from build123d import *

# Parameters (mm, degrees)
F0_R     = 12.5
F1_DEPTH = 6.5
F2_R     = 10
F3_DEPTH = 5
F4_R     = 8
F5_DEPTH = 11.501
F6_SIZE  = 0.2


with BuildPart() as f1:
    # F0 (on Top) → F1 (new body)
    with BuildSketch(Plane.XY):
        Circle(F0_R)
    extrude(amount=F1_DEPTH)

    # F2 (on face) → F3 (join)
    with BuildSketch(Plane.XY.offset(6.5)):
        Circle(F2_R)
    extrude(amount=F3_DEPTH)

    # F4 (on face) → F5 (cut, through all)
    with BuildSketch(Plane.XY.offset(11.5)):
        Circle(F4_R)
    extrude(amount=-F5_DEPTH, mode=Mode.SUBTRACT)

    # F6
    f6_edges = [f1.edges().sort_by_distance(p)[0] for p in [
        (-10, 0, 11.5),
        (-8, 0, 11.5),
        (-12.5, 0, 6.5),
        (-10, 0, 6.5),
        (-12.5, 0, 0),
        (-8, 0, 0),
    ]]
    chamfer(f6_edges, length=F6_SIZE)


solid = f1.part
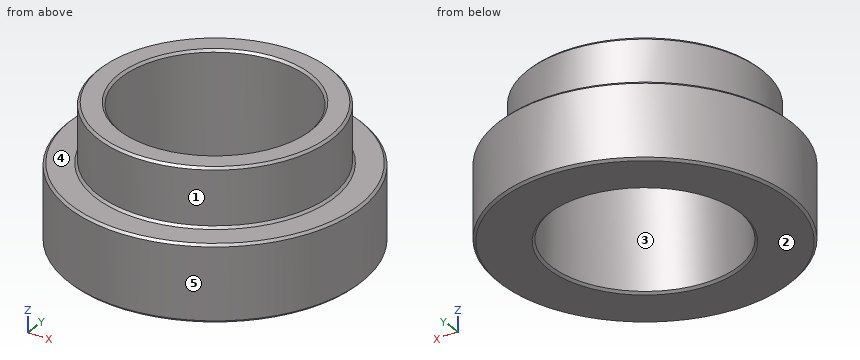
For this review, take the finished solid that the model builds, in its own axes (mm). Face numbers are marked on the shaded views. A direction names the side the tool comes from. Round coordinates to 2 decimals unless told otherwise and drop trailing zeros. Loops run counter-clockwise (first coordinate to the right, second up) from the corner with the lowest first, then second, coordinate; pieces in that order, holes last. Notation, with made-up numbers: (71.25, 22.25) - (81.25, 22.25) arc R8 ccw to (81.25, 36.25) - close; hole circle Ø11 at (-19.75, -23). An arc over 180 degrees is marked (long way). One line per item, written item: value. Start each with the question number.
Item 1: Take a section at C-C (z = 8). Give the boundary of the cut face in (x, y), plus the area to 3 significant figures.
Item 2: For the marked faces 1 and 2, list the 3-axis set-ups (+Z, -Z, +X, -X, +Y, -Y) from which the entire face can be reached by the end or side of a thin tool; tool diameter is ignored.
Item 3: For L1, parallel to Y at x = 0, z = 7; L2, parallel to Y at x = 0, z = 6.25; L3, parallel to Z at x = 8.75, y = 5.5, list the stretches that pass through material, from the lowest coordinate up.
Item 4: Take a section at D-D (z = 2.5). Give the boundary of the cut face in (x, y), plus the area to 3 significant figures.
Item 5: The part is to be moulded in two halves that separate along X. For the marked faces 3, 4 and 5, say which applies: +X half, -X half, draft (parallel to the pull), parting line (faces both ways), or undercut.
Item 6: Clearance check with flat-ended pins moving along their axes: pin 1 Ø5 at (y, z) = (-8, 3.5) entering from +X (3 decimals); pin 2 Ø6 at (x, y) = (-9, -8) entering from -Z; pin 3 Ø4 at (y, z) = (6.5, 1.5) entering from -X; pin 4 Ø4 at (x, z) = (7.5, 5.5) entering from -Y (3 decimals). State where each tip first meets the part, or that it passes through.
Item 7: Take a section at A-A (x = 0). Give the boundary of the cut face in (y, z), plus the area to 3 significant figures.
Answer below:
1. outline: circle Ø20 at (0, 0); hole circle Ø16 at (0, 0)
1. area: 113 mm2
2. face 1: +Z
2. face 2: -Z, +X, -X, +Y, -Y
3. L1: y = -10 to -8, 8 to 10
3. L2: y = -12.5 to -8, 8 to 12.5
3. L3: z = 0 to 6.5
4. outline: circle Ø25 at (0, 0); hole circle Ø16 at (0, 0)
4. area: 290 mm2
5. face 3: undercut
5. face 4: draft
5. face 5: parting line
6. pin 1: stops at x = 11.225
6. pin 2: stops at z = 0
6. pin 3: stops at x = -11.66
6. pin 4: stops at y = -11.225
7. outline: (-12.5, 0.2) - (-12.3, 0) - (-8.2, 0) - (-8, 0.2) - (-8, 11.3) - (-8.2, 11.5) - (-9.8, 11.5) - (-10, 11.3) - (-10, 6.7) - (-10.2, 6.5) - (-12.3, 6.5) - (-12.5, 6.3) - close; (8, 0.2) - (8.2, 0) - (12.3, 0) - (12.5, 0.2) - (12.5, 6.3) - (12.3, 6.5) - (10.2, 6.5) - (10, 6.7) - (10, 11.3) - (9.8, 11.5) - (8.2, 11.5) - (8, 11.3) - close
7. area: 78.3 mm2
